CAD build for the part. Positions are in the model's coordinates, mm. A direction names the side the tool comes from. Give positions to 0.01 mm unless a question says otherwise; leave off trailing zeros. Order: outer loops, then holes, each group sorted by start corner. A loop starts at its lowest first (then second) coordinate and runs counter-clockwise, first axis right, second up. Notation, with made-up numbers: M 58.25,53.25 L 109.25,53.25 A18 cw 109.25,78.25 Z; hole C -1.5,84.5 d2. An arc over 180 degrees is marked long. Put each result on its own line as item: value. Start each with the question number.
1) Pin check, flat tips, straight feed: pin 1 (2.5 mm diameter, centred on x = -7.5, y = 7.5, fed in from -Z); pin 2 (3 mm diameter, centred on x = -8, z = 0, fed in from +Y); pin 3 (2 mm diameter, centred on x = 0, z = -8, fed in from -Y); pin 4 (3 mm diameter, centred on x = 7.5, y = 7.5, fed in from -Z). Stop position of each tip, or through.
2) Cut at D-D (x = 10). Write the cut outline in (y, z) (3 decimals).
3) Drill centre lines: line 1 (X direction, y = 9.95, z = -8); line 2 (Y direction, x = -7.5, z = -6.5). Where is each one in solid material? Low to high. Write a range as [from, to].
4) Two-plate mould, pull along X, no slides. Class faces 1 (the face through (0, 0, -6)), 2 (the face through (-11, 7, 12)), 3 (the face through (5, 11.25, 2)): released by +X, released by -X, zero draft, split by the parting line, or undercut.
5) Cut at B-B (z = -4). Write the cut outline in (x, y).
6) Cut at A-A (y = 14). Write the cut outline in (x, z) (3 decimals).
7) Tool access for faces 4 (the face through (0.27, 8.21, -6.78)), 5 (the face through (0, 7, -12.5)), 6 (the face through (-9.15, 7.57, -8.44)): list every direction of +Z, -Z, +X, -X, +Y, -Y with a clear straight run to the whole face (end or side of a thin tool).
8) Cut at C-C (x = -2). Write the cut outline in (y, z).
```python
from build123d import *

# Parameters (mm, degrees)
SKETCH1_W                 = 25
SKETCH1_H                 = 25
BOSS_EXTRUDE1_DEPTH       = 15
SKETCH2_R                 = 11.125
CUT_EXTRUDE1_DEPTH        = 3.75
SKETCH3_R                 = 5.125
CUT_EXTRUDE2_DEPTH        = 12.25
M3X0_5_TAPPED_HOLE1_D     = 2.5
M3X0_5_TAPPED_HOLE1_DEPTH = 6
M3X0_5_TAPPED_HOLE1_TIP   = 0.751075774
M4X0_7_TAPPED_HOLE1_D     = 3.3
M4X0_7_TAPPED_HOLE1_DEPTH = 8
M4X0_7_TAPPED_HOLE1_TIP   = 0.991420021
CHAMFER1_SIZE             = 2


with BuildPart() as part:
    # Sketch1 → Boss-Extrude1 (new body)
    with BuildSketch(Plane(origin=(0, 0, 0), x_dir=(1, 0, 0), z_dir=(0, 1, 0))):
        Rectangle(SKETCH1_W, SKETCH1_H)
    extrude(amount=BOSS_EXTRUDE1_DEPTH)

    # Sketch2 → Cut-Extrude1 (cut)
    with BuildSketch(Plane(origin=(0, 15, 0), x_dir=(1, 0, 0), z_dir=(0, 1, 0))):
        Circle(SKETCH2_R)
    extrude(amount=-CUT_EXTRUDE1_DEPTH, mode=Mode.SUBTRACT)

    # Sketch3 → Cut-Extrude2 (cut, through all)
    with BuildSketch(Plane(origin=(0, 11.25, 0), x_dir=(1, 0, 0), z_dir=(0, 1, 0))):
        Circle(SKETCH3_R)
    extrude(amount=-CUT_EXTRUDE2_DEPTH, mode=Mode.SUBTRACT)

    # M3x0.5 Tapped Hole1
    with Locations(Plane(origin=(0, 11.25, 0), x_dir=(1, 0, 0), z_dir=(0, 1, 0))):
        with Locations((-8, 0), (8, 0), (0, 8), (0, -8)):
            Hole(M3X0_5_TAPPED_HOLE1_D / 2, depth=M3X0_5_TAPPED_HOLE1_DEPTH)
            with Locations((0, 0, -(M3X0_5_TAPPED_HOLE1_DEPTH + M3X0_5_TAPPED_HOLE1_TIP / 2))):  # 118° drill point
                Cone(0, M3X0_5_TAPPED_HOLE1_D / 2, M3X0_5_TAPPED_HOLE1_TIP, mode=Mode.SUBTRACT)

    # M4x0.7 Tapped Hole1
    with Locations(Plane(origin=(0, 0, -12.5), x_dir=(-1, 0, 0), z_dir=(0, 0, -1))):
        with Locations((-7.5, 7.5), (7.5, 7.5)):
            Hole(M4X0_7_TAPPED_HOLE1_D / 2, depth=M4X0_7_TAPPED_HOLE1_DEPTH)
            with Locations((0, 0, -(M4X0_7_TAPPED_HOLE1_DEPTH + M4X0_7_TAPPED_HOLE1_TIP / 2))):  # 118° drill point
                Cone(0, M4X0_7_TAPPED_HOLE1_D / 2, M4X0_7_TAPPED_HOLE1_TIP, mode=Mode.SUBTRACT)

    # Chamfer1
    chamfer1_edges = [part.edges().sort_by_distance(p)[0] for p in [
        (12.5, 7.5, 12.5),
        (-12.5, 7.5, 12.5),
    ]]
    chamfer(chamfer1_edges, length=CHAMFER1_SIZE)


solid = part.part
```
Solution:
1. pin 1: z = -4.26
1. pin 2: y = 11.25
1. pin 3: y = 0
1. pin 4: z = -4.41
2. outline: M 0,-12.5 L 15,-12.5 L 15,-4.875 L 11.25,-4.875 L 11.25,4.875 L 15,4.875 L 15,12.5 L 0,12.5 Z
3. line 1: [-12.5, -1.25], [1.25, 12.5]
3. line 2: [0, 5.85], [9.15, 11.25]
4. face 1: zero draft
4. face 2: released by -X
4. face 3: undercut
5. outline: M -12.5,0 L -3.2,0 L -3.2,11.25 L -10.38,11.25 L -10.38,15 L -12.5,15 Z; M 3.2,0 L 12.5,0 L 12.5,15 L 10.38,15 L 10.38,11.25 L 3.2,11.25 Z; hole C -7.5,7.5 d1.64; hole C 7.5,7.5 d1.64
6. outline: M -12.5,-12.5 L 12.5,-12.5 L 12.5,10.5 L 10.5,12.5 L -10.5,12.5 L -12.5,10.5 Z; hole C 0,0 d22.25
7. face 4: +Y
7. face 5: -Z, +X, -X, +Y, -Y
7. face 6: -Z
8. outline: M 0,-12.5 L 15,-12.5 L 15,-10.94 L 11.25,-10.94 L 11.25,-4.72 L 0,-4.72 Z; M 0,4.72 L 11.25,4.72 L 11.25,10.94 L 15,10.94 L 15,12.5 L 0,12.5 Z
